Geometry check sheet. Reference: the model listing, model coordinates, mm. Face numbers are marked on the shaded views. A direction names the side the tool comes from. Round coordinates to 2 decimals unless told otherwise and drop trailing zeros. Order: outer loops, then holes, each group sorted by start corner. A loop starts at its lowest first (then second) coordinate and runs counter-clockwise, first axis right, second up.
```python
from build123d import *

# Parameters (mm, degrees)
SKETCH1_W                                           = 104
SKETCH1_H                                           = 104
BOSS_EXTRUDE1_DEPTH                                 = 10
FILLET1_R                                           = 5
CUT_EXTRUDE1_DEPTH                                  = 11
CIRPATTERN1_COUNT                                   = 4
CBORE_FOR_12_BINDING_HEAD_MACHINE_SCREW_D           = 4.8006
CBORE_FOR_12_BINDING_HEAD_MACHINE_SCREW_CBORE_D     = 9.525
CBORE_FOR_12_BINDING_HEAD_MACHINE_SCREW_CBORE_DEPTH = 2.921
FILLET3_R                                           = 2
CIRPATTERN5_COUNT                                   = 4


with BuildPart() as part:
    # Sketch1 → Boss-Extrude1 (new body)
    with BuildSketch(Plane(origin=(0, 0, 0), x_dir=(1, 0, 0), z_dir=(0, 1, 0))):
        Rectangle(SKETCH1_W, SKETCH1_H)
        Polygon((-42, 47), (-42, 37), (-47, 37), (-47, 5), (-35, 5), (-5, 35), (-5, 47), align=None, mode=Mode.SUBTRACT)
        Polygon((-32.928932188, 0), (0, 32.928932188), (32.928932188, 0), (0, -32.928932188), align=None, mode=Mode.SUBTRACT)
        Polygon((5, 47), (5, 35), (35, 5), (47, 5), (47, 42), (37, 42), (37, 47), align=None, mode=Mode.SUBTRACT)
        Polygon((47, -5), (35, -5), (5, -35), (5, -47), (42, -47), (42, -37), (47, -37), align=None, mode=Mode.SUBTRACT)
        Polygon((-5, -47), (-5, -35), (-35, -5), (-47, -5), (-47, -42), (-37, -42), (-37, -47), align=None, mode=Mode.SUBTRACT)
    extrude(amount=BOSS_EXTRUDE1_DEPTH)

    # Fillet1
    fillet1_edges = [part.edges().sort_by_distance(p)[0] for p in [
        (-5, 5, -35),
        (-5, 5, -47),
        (-42, 5, -47),
        (-47, 5, -5),
        (-35, 5, -5),
        (-32.928932188, 5, 0),
        (0, 5, 32.928932188),
        (32.928932188, 5, 0),
        (0, 5, -32.928932188),
        (5, 5, -35),
        (35, 5, -5),
        (47, 5, -5),
        (47, 5, -42),
        (5, 5, -47),
        (35, 5, 5),
        (5, 5, 35),
        (5, 5, 47),
        (42, 5, 47),
        (47, 5, 5),
        (-5, 5, 35),
        (-35, 5, 5),
        (-47, 5, 5),
        (-47, 5, 42),
        (-5, 5, 47),
    ]]
    fillet(fillet1_edges, radius=FILLET1_R)

    # Sketch2 → Cut-Extrude1 (cut, through all)
    with BuildSketch(Plane(origin=(0, 10, 0), x_dir=(1, 0, 0), z_dir=(0, 1, 0))):
        Polygon((-52, 52), (-42, 52), (-42, 50), (-50, 50), (-50, 42), (-52, 42), align=None)
    cut_extrude1 = extrude(amount=-CUT_EXTRUDE1_DEPTH, mode=Mode.SUBTRACT)

    # CirPattern1: Cut-Extrude1 ×4 about axis
    cirpattern1_axis = Axis((0, 0, 0), (0, 1, 0))
    for i in range(1, CIRPATTERN1_COUNT):
        add(cut_extrude1.rotate(cirpattern1_axis, i * 360 / CIRPATTERN1_COUNT), mode=Mode.SUBTRACT)

    # CBORE for #12 Binding Head Machine Screw1 (through all)
    with Locations(Plane(origin=(0, 10, 0), x_dir=(1, 0, 0), z_dir=(0, 1, 0))):
        with Locations((0, 36.5), (-36.5, 0), (0, -36.5), (36.5, 0)):
            CounterBoreHole(CBORE_FOR_12_BINDING_HEAD_MACHINE_SCREW_D / 2, CBORE_FOR_12_BINDING_HEAD_MACHINE_SCREW_CBORE_D / 2, CBORE_FOR_12_BINDING_HEAD_MACHINE_SCREW_CBORE_DEPTH)

    # Fillet3
    fillet3_edges = [part.edges().sort_by_distance(p)[0] for p in [
        (-42, 5, -37),
        (-47, 5, -37),
        (37, 5, -42),
        (37, 5, -47),
        (42, 5, 37),
        (47, 5, 37),
        (-37, 5, 42),
        (-37, 5, 47),
    ]]
    fillet(fillet3_edges, radius=FILLET3_R)

    # Sketch9 → #10-24 Tapped Hole1 (revolve, cut)
    with BuildSketch(Plane(origin=(50, 5, -47), x_dir=(0, 0, -1), z_dir=(0, 1, 0))):
        Polygon((0, 0), (0, 21.140824014), (1.89865, 20), (1.89865, 0), align=None)
    f_10_24_tapped_hole1 = revolve(axis=Axis((56.35, 5, -47), (-1, 0, 0)), mode=Mode.SUBTRACT)

    # CirPattern5: #10-24 Tapped Hole1 ×4 about axis
    cirpattern5_axis = Axis((0, 10.5, 0), (0, -1, 0))
    for i in range(1, CIRPATTERN5_COUNT):
        add(f_10_24_tapped_hole1.rotate(cirpattern5_axis, i * 360 / CIRPATTERN5_COUNT), mode=Mode.SUBTRACT)


solid = part.part
```
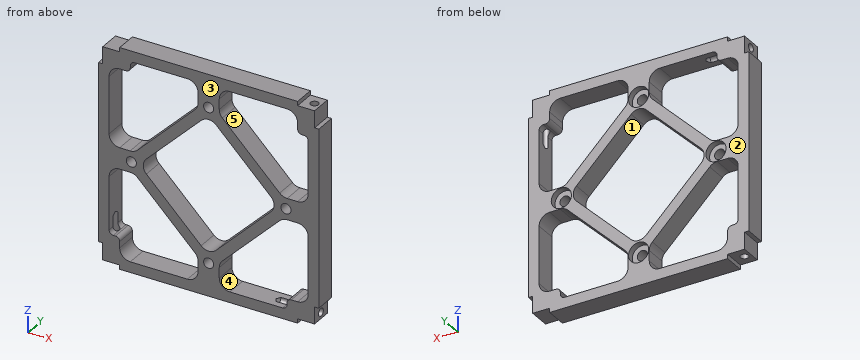
(1) Set-up check for the marked faces 1 and 2: record each of +Z, -Z, +X, -X, +Y, -Y from which the full face is reachable in a straight line by a thin tool's end or side.
Returned:
face 1: +Y, -Y
face 2: +Z, -Z, +X, -X, +Y
(2) Sectioned sample at B-B, the plane x = 0. Record the cut outline in (y, z).
Returned:
outline: (0, -52) - (10, -52) - (10, -41.26) - (7.08, -41.26) - (7.08, -38.9) - (0, -38.9) - close; (0, -34.1) - (7.08, -34.1) - (7.08, -31.74) - (10, -31.74) - (10, -30.86) - (0, -30.86) - close; (0, 30.86) - (10, 30.86) - (10, 31.74) - (7.08, 31.74) - (7.08, 34.1) - (0, 34.1) - close; (0, 38.9) - (7.08, 38.9) - (7.08, 41.26) - (10, 41.26) - (10, 52) - (0, 52) - close
(3) Depth check by flat-ended pin: P1, Ø2, axis at x = 50.5, y = 4, coming from the +Z side; P2, Ø0.6, axis at y = 4.5, z = 51, coming from the -X side; P3, Ø0.8, axis at y = 7.5, z = -44.5, coming from the -X side. Enter the tip coordinate at first touch or a pass-through.
Returned:
P1: stops at z = 50
P2: stops at x = -42
P3: stops at x = -50
(4) Material ranges on line 1 (Z direction, x = 0, y = 3.75); line 2 (X direction, y = 6.5, z = 46.5); line 3 (X direction, y = 0.75, z = -18), recorded low to high.
Returned:
line 1: z = -52 to -38.9, -34.1 to -30.86, 30.86 to 34.1, 38.9 to 52
line 2: x = -7.82 to 7.82, 39.18 to 45.84, 48.16 to 50
line 3: x = -52 to -47, -22 to -14.93, 14.93 to 22, 47 to 52
(5) Sectioned sample at A-A, the plane z = 0. Record the cut outline in (x, y), and give its area (3 significant figures).
Returned:
outline: (-52, 0) - (-38.9, 0) - (-38.9, 7.08) - (-41.26, 7.08) - (-41.26, 10) - (-52, 10) - close; (-34.1, 0) - (-30.86, 0) - (-30.86, 10) - (-31.74, 10) - (-31.74, 7.08) - (-34.1, 7.08) - close; (30.86, 0) - (34.1, 0) - (34.1, 7.08) - (31.74, 7.08) - (31.74, 10) - (30.86, 10) - close; (38.9, 0) - (52, 0) - (52, 10) - (41.26, 10) - (41.26, 7.08) - (38.9, 7.08) - close
area: 299 mm2
(6) Sectioned sample at C-C, the plane x = -19.5. Record the cut outline in (y, z), and give its area (3 significant figures).
Returned:
outline: (0, -52) - (10, -52) - (10, -47) - (0, -47) - close; (0, -20.5) - (10, -20.5) - (10, -13.43) - (0, -13.43) - close; (0, 13.43) - (10, 13.43) - (10, 20.5) - (0, 20.5) - close; (0, 47) - (10, 47) - (10, 52) - (0, 52) - close
area: 241 mm2
(7) Draft check along Z on the marked faces 3, 4 and 5. Enter one of: released by +Z, released by -Z, zero draft, split by the parting line, or undercut.
Returned:
face 3: zero draft
face 4: undercut
face 5: undercut
